The drawing under review shows one solid part. Ordinate dimensions are in mm from its lowest x, y, z. Coordinates: 2 decimals unless noted, no trailing zeros. Loops run counter-clockwise (first coordinate to the right, second up) from the corner with the lowest first, then second, coordinate; pieces in that order, holes last. Notation, with made-up numbers: (-26.75, 45) -> (-5.75, 45) arc R20 cw to (-5.75, 83) -> close; hole circle Ø7 at (-12.5, -15). An arc over 180 degrees is marked (long way). Use a Markdown table: item, result.
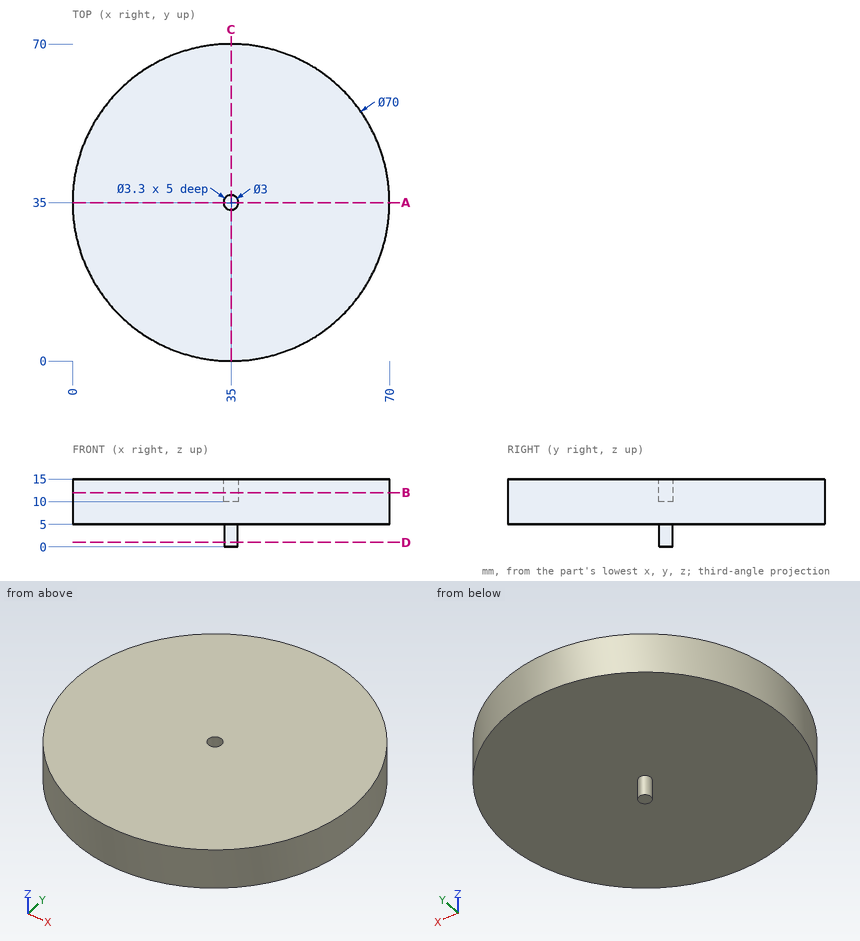
(1) For pin 1 Ø1 at (y, z) = (18.5, 8.5) entering from +X; pin 2 Ø3 at (x, z) = (54, 13.5) entering from -Y; pin 3 Ø4 at (y, z) = (41, 5) entering from +X, all flat-tipped, find the tip position at first contact; note any pin that passes through.
Found:
| item | result |
|---|---|
| pin 1 | stops at x = 66.13 |
| pin 2 | stops at y = 4.69 |
| pin 3 | stops at x = 69.77 |
(2) Take a section at D-D on z = 1. Write out the cut boundary in (x, y).
Found:
| item | result |
|---|---|
| outline | circle Ø3 at (35, 35) |
(3) For line 1 along Y through (x, z) = (35, 13.85); line 2 along Z through (x, y) = (31, 32.5); line 3 along Y through (x, z) = (51, 13.25), list the stretches that pass through material, from the lowest coordinate up.
Found:
| item | result |
|---|---|
| line 1 | y = 0 to 33.35, 36.65 to 70 |
| line 2 | z = 5 to 15 |
| line 3 | y = 3.87 to 66.13 |
(4) Take a section at A-A on y = 35. Write out the cut boundary in (x, z), plus the area to 4 significant figures.
Found:
| item | result |
|---|---|
| outline | (0, 5) -> (33.5, 5) -> (33.5, 0) -> (36.5, 0) -> (36.5, 5) -> (70, 5) -> (70, 15) -> (36.65, 15) -> (36.65, 10) -> (33.35, 10) -> (33.35, 15) -> (0, 15) -> close |
| area | 698.5 mm^2 |
(5) Take a section at B-B on z = 12. Write out the cut boundary in (x, y).
Found:
| item | result |
|---|---|
| outline | circle Ø70 at (35, 35); hole circle Ø3.3 at (35, 35) |
